Part model, mm, in its own coordinate system. A direction names the side the tool comes from. Round coordinates to 2 decimals unless told otherwise and drop trailing zeros. Write each loop counter-clockwise with the first axis right and the second up, starting at its lowest first coordinate (ties: lowest second). Pieces come first, ordered by that corner, then holes.
1) Saw through at B-B on x = 10. Write the cut outline in (y, z), and give its area (3 significant figures).
2) Drill centre lines: L1, parallel to Y at x = -331.5, z = -27; L2, parallel to Z at x = -287, y = 581; L3, parallel to X at y = -138, z = -31.5. Where is each one in solid material? Low to high.
3) Which spindle directions (+Z, -Z, +X, -X, +Y, -Y) get a long thin tool onto all of the face, cutting with end or side? Do faces 5 (the flat face through (-5, -583, -18)), 6 (the flat face through (-406, 3, 0)), 7 (the flat face through (-260, -7.5, 28)). Say none if no direction does.
4) Pull direction X, two halves, no side cores. Call faces 1 (the flat face through (379.8, -8, -18)), 2 (the flat face through (5, 583, -18)), 3 (the flat face through (-5, 8, 0)), 4 (the flat face through (-379.8, 8, -18)): +X half, -X half, draft (parallel to the pull), parting line (faces both ways), or undercut.
5) Saw through at A-A on y = -130.5. Write the cut outline in (x, z), and give its area (3 significant figures).
6) Flat gauge pins, fed straight in: pin 1 (15 mm diameter, centred on y = -3, z = 28.5, fed in from +X); pin 2 (19 mm diameter, centred on x = -287.3, z = -25, fed in from -Y); pin 3 (5 mm diameter, centred on x = 219, z = -11, fed in from +Y); pin 4 (6 mm diameter, centred on x = 7, z = 8.5, fed in from +Y). Where does each tip first touch, or does it go through?
Autodesk Inventor part; units mm, degrees
ref_plane "YZ Plane" through (0, 0, 0) normal (1, 0, 0) x (0, 1, 0)
ref_plane "XZ Plane" through (0, 0, 0) normal (0, 1, 0) x (-1, 0, 0)
ref_plane "XY Plane" through (0, 0, 0) normal (0, 0, 1) x (1, 0, 0)
sketch "Sketch1" plane through (0, 0, 0) normal (0, 0, 1) x (1, 0, 0)
  line L0 (-379.8, -583) -> (379.8, -583)
  line L1 (379.8, -583) -> (379.8, 583)
  line L2 (379.8, 583) -> (-379.8, 583)
  line L3 (-379.8, 583) -> (-379.8, -583)
  line L4 (-379.8, -583) -> (379.8, 583) construction
  line L5 (379.8, -583) -> (-379.8, 583) construction
  point P0 (0, 0)
  dimension "d0" = 759.6
  dimension "d1" = 1166
extrude "Extrusion1" add sketch "Sketch1" along normal blind 3
sketch "Sketch2" plane through (0, 0, 3) normal (0, 0, 1) x (1, 0, 0)
  line L0 (379.8, 583) -> (-379.8, 583)
  line L1 (379.8, -583) -> (379.8, 583)
  line L2 (-379.8, -583) -> (379.8, -583)
  line L3 (-379.8, 583) -> (-379.8, -583)
  line L4 (-376.8, 580) -> (376.8, 580)
  line L5 (376.8, 580) -> (376.8, -580)
  line L6 (376.8, -580) -> (-376.8, -580)
  line L7 (-376.8, -580) -> (-376.8, 580)
  point P0 (0, 0)
  dimension "d4" = 3
extrude "Extrusion2" add sketch "Sketch2" against normal blind 38
sketch "Sketch3" plane through (0, 0, 3) normal (0, 0, 1) x (1, 0, 0)
  line L0 (-299.8, -7.5) -> (-274.8, -7.5)
  line L1 (-274.8, -7.5) -> (-274.8, 7.5)
  line L2 (-274.8, 7.5) -> (-299.8, 7.5)
  line L3 (-299.8, 7.5) -> (-299.8, -7.5)
  line L4 (-299.8, -7.5) -> (-274.8, 7.5) construction
  line L5 (-274.8, -7.5) -> (-299.8, 7.5) construction
  line L6 (-379.8, 583) -> (-379.8, -583)
  point P0 (0, 0)
  point P1 (-287.3, 0)
  dimension "d7" = 25
  dimension "d8" = 15
  dimension "d9" = 80
extrude "Extrusion3" add sketch "Sketch3" along normal blind 35
sketch "Sketch4" plane through (-274.8, -7.5, 3) normal (1, 0, 0) x (0, 0, -1)
  line L0 (-35, 0) -> (-35, 15)
  line L1 (-35, 15) -> (-20, 15)
  line L2 (-20, 15) -> (-20, 0)
  line L3 (-20, 0) -> (-35, 0)
  line L4 (-35, 0) -> (-35, 15)
  point P0 (3, 7.5)
  dimension "d12" = 15
  dimension "d13" = 15
extrude "Extrusion4" add sketch "Sketch4" along normal blind 80
draft "FaceDraft2" angle 1 pull direction (1, 0, 0) faces at (-256.4667, 7.5, 33) fixed edges at (-274.8, 7.5, 13)
sketch "Sketch5" plane through (-379.8, 583, 3) normal (0, 1, 0) x (1, 0, 0)
  line L0 (80, 0) -> (80, -35) construction
  line L1 (105, 0) -> (105, -20) construction
  line L2 (80, 0) -> (105, 0) construction
  line L3 (759.6, 0) -> (0, 0)
  line L4 (92.5, 0) -> (92.5, 56) construction
  circle A0 centre (92.5, 28) radius 6
  line L5 (0, 38) -> (759.6, 38)
  point P0 (379.8, 3)
  dimension "d18" = 12.5
  dimension "d19" = 12
  dimension "d20" = 10
extrude "Extrusion5" cut sketch "Sketch5" against normal through all
sketch "Sketch7" plane through (0, 0, 3) normal (0, 0, 1) x (1, 0, 0)
  line L0 (379.8, 583) -> (-379.8, 583)
  line L1 (-379.8, 583) -> (-379.8, -583)
  line L2 (379.8, -583) -> (379.8, 583)
  line L3 (-379.8, -583) -> (379.8, -583)
  line L4 (-419.8, 623) -> (419.8, 623)
  line L5 (419.8, 623) -> (419.8, -623)
  line L6 (419.8, -623) -> (-419.8, -623)
  line L7 (-419.8, -623) -> (-419.8, 623)
  point P0 (0, 0)
  dimension "d26" = 40
extrude "Extrusion7" add sketch "Sketch7" against normal blind 3
properties part number "EnclosureDoor" material "Steel, Galvanized"
Completed:
1. outline: (-623, 0) - (-583, 0) - (-583, -35) - (-580, -35) - (-580, 0) - (580, 0) - (580, -35) - (583, -35) - (583, 0) - (623, 0) - (623, 3) - (-623, 3) - close
1. area: 3,950 mm2
2. L1: y = -583 to -580, 580 to 583
2. L2: z = -35 to -30.99, -19.01 to 3
2. L3: x = -379.8 to -376.8, 376.8 to 379.8
3. face 5: -Z, +X, -X, -Y
3. face 6: -Z
3. face 7: +Z, +X, -X, -Y
4. face 1: +X half
4. face 2: draft
4. face 3: undercut
4. face 4: -X half
5. outline: (-419.8, 0) - (-379.8, 0) - (-379.8, -35) - (-376.8, -35) - (-376.8, 0) - (376.8, 0) - (376.8, -35) - (379.8, -35) - (379.8, 0) - (419.8, 0) - (419.8, 3) - (-419.8, 3) - close
5. area: 2,730 mm2
6. pin 1: stops at x = -194.8
6. pin 2: stops at y = -583
6. pin 3: stops at y = 583
6. pin 4: passes through
